The model under review builds one solid part; all positions refer to its coordinate system, in mm. A direction names the side the tool comes from. Give positions to 0.01 mm unless a question says otherwise; leave off trailing zeros. Loops run counter-clockwise (first coordinate to the right, second up) from the corner with the lowest first, then second, coordinate; pieces in that order, holes last. Notation, with made-up numbers: (18, 71.5) -> (24, 71.5) arc R14 cw to (24, 85.5) -> close; hole circle Ø9 at (38.25, 61). An arc over 180 degrees is marked (long way). Write each question's results on one line, items separated by ' | '. Start each with the question number.
Q1. Mouldability with a two-part tool opening along X and no side actions: class faces 4 (the face through (-10, 62, -6)), 5 (the face through (4.27, 61.62, -5.33)), 6 (the face through (0.1, 125, 2.4)) as released by +X, released by -X, zero draft, split by the parting line, or undercut.
Q2. Insertion check: pin 1 Ø1.4 at (x, y) = (1, 90.5) entering from +Z (3 decimals); pin 2 Ø2.5 at (x, z) = (0, 0) entering from -Y; pin 3 Ø5 at (y, z) = (64.5, 0.5) entering from -X; pin 4 Ø2.5 at (x, y) = (0, 45.5) entering from -Z (3 decimals). Each pin has a flat end and moves straight along its axis. Give the tip position at first contact, or say it passes through.
Q3. We need section B-B (x = 0). Write out the cut boundary in (y, z) (3 decimals), plus the area to 3 significant figures.
Q4. We need section A-A (z = 0). Write out the cut boundary in (x, y) (3 decimals), plus the area to 3 significant figures.
Q5. Wall thickness on L1, parallel to X at y = 43.5, z = 0 (3 decimals); L2, parallel to Z at x = -5, y = 76: over which ranges is each line inside the solid? List them lowest first. Write a range as [from, to].
Q6. Machinability: for faces 1 (the face through (3.655, 62, 0)), 2 (the face through (0, 62, -3.655)), 3 (the face through (4.27, 61.62, 5.33)), which of the approach directions +Z, -Z, +X, -X, +Y, -Y give a long, thin tool a straight path to every point of the face, cutting with its end or side? Answer none if there is none.
Autodesk Inventor part; units mm, degrees
ref_plane "YZ Plane" through (0, 0, 0) normal (1, 0, 0) x (0, 1, 0)
ref_plane "XZ Plane" through (0, 0, 0) normal (0, 1, 0) x (-1, 0, 0)
ref_plane "XY Plane" through (0, 0, 0) normal (0, 0, 1) x (1, 0, 0)
sketch "Sketch1" plane through (0, 0, 0) normal (0, 1, 0) x (-1, 0, 0)
  line L0 (0, -14) -> (0, 14)
  line L1 (-14, 0) -> (14, 0)
  line L2 (14, 0) -> (-14, 0)
  line L3 (0, -14) -> (0, 14)
  line L4 (2.5943, 3.655) -> (-2.5943, 3.655)
  line L5 (-3.655, 2.5943) -> (-3.655, -2.5943)
  line L6 (-2.5943, -3.655) -> (2.5943, -3.655)
  line L7 (3.655, -2.5943) -> (3.655, 2.5943)
  line L8 (-3.655, 3.655) -> (3.655, -3.655) construction
  line L9 (10, 10) -> (10, 2.63)
  line L10 (10, 2.63) -> (8.5, 2.63)
  line L11 (10, 10) -> (2.63, 10)
  line L12 (2.63, 10) -> (2.63, 8.5)
  line L13 (-10, 10) -> (-2.63, 10)
  line L14 (-2.63, 10) -> (-2.63, 8.5)
  line L15 (-10, 8.5) -> (-10, 10)
  line L16 (-10, 10) -> (-8.5, 10)
  line L17 (-8.5, 2.63) -> (-10, 2.63)
  line L18 (-10, 2.63) -> (-10, 10)
  line L19 (-10, -10) -> (-8.5, -10)
  line L20 (-8.5, -2.63) -> (-10, -2.63)
  line L21 (-10, -2.63) -> (-10, -10)
  line L22 (-10, -10) -> (-2.63, -10)
  line L23 (-2.63, -10) -> (-2.63, -8.5)
  line L24 (-10, -8.5) -> (-10, -10)
  line L25 (10, -10) -> (8.5, -10)
  line L26 (8.5, -2.63) -> (10, -2.63)
  line L27 (10, -2.63) -> (10, -10)
  line L28 (10, -10) -> (2.63, -10)
  line L29 (2.63, -10) -> (2.63, -8.5)
  line L30 (10, -8.5) -> (10, -10)
  circle A0 centre (0, 0) radius 2.095
  line L31 (5.995, -10) -> (2.63, -10)
  line L32 (-2.63, -10) -> (-5.995, -10)
  line L33 (10, -10) -> (2.63, -10)
  line L34 (-2.63, -10) -> (-10, -10)
  line L35 (10, -5.995) -> (10, -2.63)
  line L36 (10, 2.63) -> (10, 5.995)
  line L37 (10, 10) -> (10, 2.63)
  line L38 (10, -2.63) -> (10, -10)
  line L39 (-5.995, 10) -> (-2.63, 10)
  line L40 (2.63, 10) -> (5.995, 10)
  line L41 (-10, 10) -> (-2.63, 10)
  line L42 (2.63, 10) -> (10, 10)
  line L43 (-10, 5.995) -> (-10, 2.63)
  line L44 (-10, -2.63) -> (-10, -5.995)
  line L45 (-10, -10) -> (-10, -2.63)
  line L46 (-10, 2.63) -> (-10, 10)
  line L47 (-2.63, -8.5) -> (-5.995, -8.5)
  line L48 (-8.5, -5.995) -> (-8.5, -2.63)
  line L49 (-8.5, -5.995) -> (-7.0557, -5.995)
  line L50 (-5.995, -8.5) -> (-5.995, -7.0557)
  line L51 (-5.995, 7.0557) -> (-5.995, 8.5)
  line L52 (2.63, 8.5) -> (5.995, 8.5)
  line L53 (8.5, 2.63) -> (8.5, 5.995)
  line L54 (8.5, 5.995) -> (7.0557, 5.995)
  line L55 (5.995, 8.5) -> (5.995, 7.0557)
  line L56 (2.63, -8.5) -> (5.995, -8.5)
  line L57 (9.5607, -8.5) -> (10, -8.5)
  line L58 (8.5, -10) -> (8.5, -9.5607)
  line L59 (8.5, -5.995) -> (8.5, -2.63)
  line L60 (7.0557, -5.995) -> (8.5, -5.995)
  line L61 (5.995, -7.0557) -> (5.995, -8.5)
  line L62 (3.655, 3.655) -> (-0.5303, -0.5303) construction
  line L63 (-1.4814, -1.4814) -> (-3.655, -3.655) construction
  line L64 (-8.5, 10) -> (-8.5, 9.5607)
  line L65 (-8.5, 5.995) -> (-8.5, 2.63)
  line L66 (-2.63, 8.5) -> (-5.995, 8.5)
  line L67 (-9.5607, 8.5) -> (-10, 8.5)
  line L68 (-7.0557, 5.995) -> (-8.5, 5.995)
  line L69 (-3.655, 2.5943) -> (-7.0557, 5.995)
  line L70 (-2.5943, 3.655) -> (-5.995, 7.0557)
  line L71 (5.995, 7.0557) -> (2.5943, 3.655)
  line L72 (7.0557, 5.995) -> (3.655, 2.5943)
  line L73 (7.0557, -5.995) -> (3.655, -2.5943)
  line L74 (5.995, -7.0557) -> (2.5943, -3.655)
  line L75 (-2.5943, -3.655) -> (-5.995, -7.0557)
  line L76 (-3.655, -2.5943) -> (-7.0557, -5.995)
  dimension "d26" = 4.19
  dimension "d0" = 20
  dimension "d1" = 20
  dimension "d2" = 7.31
  dimension "d3" = 7.31
  dimension "d4" = 20
  dimension "d5" = 11.99
  dimension "d6" = 11.99
  dimension "d11" = 7.37
  dimension "d12" = 1.5
  dimension "d13" = 7.37
  dimension "d14" = 1.5
  dimension "d15" = 7.37
  dimension "d16" = 1.5
  dimension "d17" = 7.37
  dimension "d18" = 1.5
  dimension "d19" = 7.37
  dimension "d20" = 7.37
  dimension "d21" = 1.5
  dimension "d22" = 1.5
  dimension "d23" = 7.37
  dimension "d24" = 7.37
  dimension "d25" = 1.5
extrude "Extrusion1" add sketch "Sketch1" along normal blind 125 contours L6 L75 L50 L47 L23 L22 L19 L21 L20 L48 L49 L76 L5 L1 A0 L0 | L0 A0 L1 L7 L73 L60 L59 L26 L27 L25 L28 L29 L56 L61 L74 L6 | L1 L5 L69 L68 L65 L17 L18 L15 L13 L14 L66 L51 L70 L4 L0 A0 | A0 L0 L4 L71 L55 L52 L12 L11 L9 L10 L53 L54 L72 L7 L1
fillet "Fillet1" radius 0.5 20 edges at (10, 62.5, 10) (2.63, 62.5, 10) (-2.63, 62.5, 10) (-2.63, 62.5, 8.5) (10, 62.5, 2.63) (8.5, 62.5, 2.63) (10, 62.5, -2.63) (8.5, 62.5, -2.63) (10, 62.5, -10) (2.63, 62.5, -8.5) (-2.63, 62.5, -10) (-2.63, 62.5, -8.5) (2.63, 62.5, -10) (-10, 62.5, -10) (-8.5, 62.5, -2.63) (-10, 62.5, -2.63) (-8.5, 62.5, 2.63) (-10, 62.5, 2.63) (-10, 62.5, 10) (2.63, 62.5, 8.5)
fillet "Fillet2" radius 0.75 24 edges at (-7.0557, 62.5, 5.995) (-3.655, 62.5, 2.5943) (-8.5, 62.5, -5.995) (-7.0557, 62.5, -5.995) (-5.995, 62.5, -8.5) (3.655, 62.5, -2.5943) (7.0557, 62.5, -5.995) (-2.5943, 62.5, 3.655) (-5.995, 62.5, 7.0557) (3.655, 62.5, 2.5943) (7.0557, 62.5, 5.995) (8.5, 62.5, 5.995) (8.5, 62.5, -5.995) (2.5943, 62.5, 3.655) (5.995, 62.5, 7.0557) (5.995, 62.5, 8.5) (-5.995, 62.5, 8.5) (-8.5, 62.5, 5.995) (2.5943, 62.5, -3.655) (5.995, 62.5, -7.0557) (5.995, 62.5, -8.5) (-5.995, 62.5, -7.0557) (-2.5943, 62.5, -3.655) (-3.655, 62.5, -2.5943)
properties part number "pro125mm"
Output:
1) face 4: released by -X | face 5: undercut | face 6: zero draft
2) pin 1: z = 3.655 | pin 2: through | pin 3: x = -9.98 | pin 4: z = -3.655
3) outline: (0, -3.655) -> (125, -3.655) -> (125, -2.095) -> (0, -2.095) -> close; (0, 2.095) -> (125, 2.095) -> (125, 3.655) -> (0, 3.655) -> close | area: 390 mm2
4) outline: (-3.655, 0) -> (-2.095, 0) -> (-2.095, 125) -> (-3.655, 125) -> close; (2.095, 0) -> (3.655, 0) -> (3.655, 125) -> (2.095, 125) -> close | area: 390 mm2
5) L1: [-3.655, -2.095], [2.095, 3.655] | L2: [-10, -8.5], [-6.06, -3.94], [3.94, 6.06], [8.5, 10]
6) face 1: +X, +Y, -Y | face 2: -Z, +Y, -Y | face 3: +Y, -Y
